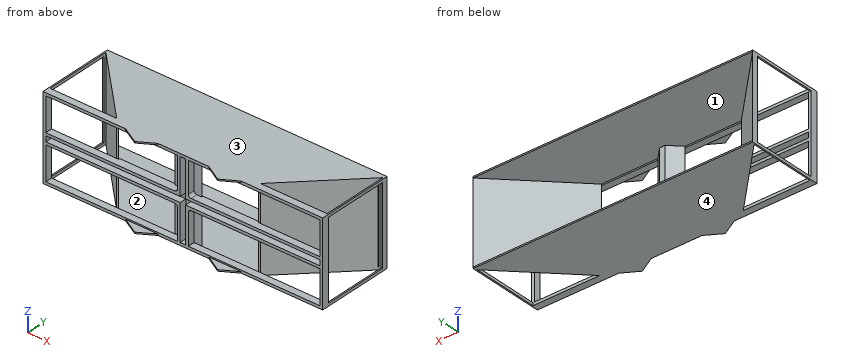
from build123d import *

# Parameters (mm, degrees)
BOSS_EXTRUDE1_DEPTH      = 10
BOSS_EXTRUDE1_DEPTH_BACK = 15
SKETCH1_W                = 1016
SKETCH1_H                = 304.8
SKETCH1_W_2              = 996
SKETCH1_H_2              = 284.8
BOSS_EXTRUDE2_DEPTH      = 10
BOSS_EXTRUDE2_DEPTH_BACK = 15
BOSS_EXTRUDE3_DEPTH      = 152.4
BOSS_EXTRUDE3_DEPTH_BACK = 152.4
SKETCH4_W                = 507.049279033
SKETCH4_H                = 40
BOSS_EXTRUDE7_DEPTH      = 5
SKETCH5_W                = 284.8
SKETCH5_H                = 234
CUT_EXTRUDE1_DEPTH       = 15
SKETCH6_W                = 284.8
SKETCH6_H                = 234
CUT_EXTRUDE2_DEPTH       = 15
BOSS_EXTRUDE8_DEPTH      = 304.8
BOSS_EXTRUDE9_DEPTH      = 5
BOSS_EXTRUDE10_DEPTH     = 5
BOSS_EXTRUDE11_DEPTH     = 5
BOSS_EXTRUDE12_DEPTH     = 5


with BuildPart() as part:
    # Sketch1 → Boss-Extrude1 (new, two sides: drawn at the far end of the back side and taken through both)
    with BuildSketch(Plane(origin=(0, 0, 0), x_dir=(1, 0, 0), z_dir=(0, 1, 0)).offset(-BOSS_EXTRUDE1_DEPTH_BACK)):
        Rectangle(SKETCH1_W, SKETCH1_H)
        Rectangle(SKETCH1_W_2, SKETCH1_H_2, mode=Mode.SUBTRACT)
    extrude(amount=BOSS_EXTRUDE1_DEPTH + BOSS_EXTRUDE1_DEPTH_BACK)

    # Sketch2 → Boss-Extrude2 (add, two sides: drawn at the far end of the back side and taken through both)
    with BuildSketch(Plane(origin=(0, 0, 0), x_dir=(1, 0, 0), z_dir=(0, 1, 0)).offset(-BOSS_EXTRUDE2_DEPTH_BACK)):
        with BuildLine():
            Line((-498, 20), (-30, 20))
            ThreePointArc((-30, 20), (-22.928932188, 22.928932188), (-20, 30))
            Line((-20, 30), (-20, 142.4))
            Line((-20, 142.4), (-10, 142.4))
            Line((-10, 142.4), (-10, 20))
            Line((-10, 20), (-10, 10))
            Line((-10, 10), (-498, 10))
            Line((-498, 10), (-498, 20))
        make_face()
        with BuildLine():
            Line((498, 20), (498, 10))
            Line((498, 10), (10, 10))
            Line((10, 10), (10, 20))
            Line((10, 20), (10, 142.4))
            Line((10, 142.4), (20, 142.4))
            Line((20, 142.4), (20, 30))
            ThreePointArc((20, 30), (22.928932188, 22.928932188), (30, 20))
            Line((30, 20), (498, 20))
        make_face()
        with BuildLine():
            Line((-498, -10), (-10, -10))
            Line((-10, -10), (-10, -20))
            Line((-10, -20), (-10, -142.4))
            Line((-10, -142.4), (-20, -142.4))
            Line((-20, -142.4), (-20, -30))
            ThreePointArc((-20, -30), (-22.928932188, -22.928932188), (-30, -20))
            Line((-30, -20), (-498, -20))
            Line((-498, -20), (-498, -10))
        make_face()
        with BuildLine():
            Line((30, -20), (498, -20))
            Line((498, -20), (498, -10))
            Line((498, -10), (10, -10))
            Line((10, -10), (10, -20))
            Line((10, -20), (10, -142.4))
            Line((10, -142.4), (20, -142.4))
            Line((20, -142.4), (20, -30))
            ThreePointArc((20, -30), (22.928932188, -22.928932188), (30, -20))
        make_face()
    extrude(amount=BOSS_EXTRUDE2_DEPTH + BOSS_EXTRUDE2_DEPTH_BACK)

    # Sketch3 → Boss-Extrude3 (add, two sides: drawn at the far end of the back side and taken through both)
    with BuildSketch(Plane.XY.offset(-BOSS_EXTRUDE3_DEPTH_BACK)):
        Polygon((-508, 10), (-508, 264), (-254, 10), (-261.071067812, 10), (-503, 251.928932188), (-503, 10), align=None)
        Polygon((261.071067812, 10), (254, 10), (508, 264), (508, 10), (503, 10), (503, 251.928932188), align=None)
    extrude(amount=BOSS_EXTRUDE3_DEPTH + BOSS_EXTRUDE3_DEPTH_BACK)

    # Sketch4 → Boss-Extrude7 (add)
    with BuildSketch(Plane(origin=(0, 10, 0), x_dir=(1, 0, 0), z_dir=(0, 1, 0))):
        with Locations((-0.42499269, 0)):
            Rectangle(SKETCH4_W, SKETCH4_H)
    extrude(amount=BOSS_EXTRUDE7_DEPTH)

    # Sketch5 → Cut-Extrude1 (cut)
    with BuildSketch(Plane(origin=(508, 0, 0), x_dir=(0, 0, -1), z_dir=(1, 0, 0))):
        with Locations((0, 127)):
            Rectangle(SKETCH5_W, SKETCH5_H)
    extrude(amount=-CUT_EXTRUDE1_DEPTH, mode=Mode.SUBTRACT)

    # Sketch6 → Cut-Extrude2 (cut)
    with BuildSketch(Plane.ZY.offset(508)):
        with Locations((0, 127)):
            Rectangle(SKETCH6_W, SKETCH6_H)
    extrude(amount=-CUT_EXTRUDE2_DEPTH, mode=Mode.SUBTRACT)

    # Sketch7 → Boss-Extrude8 (add)
    with BuildSketch(Plane(origin=(0, 0, -152.4), x_dir=(-1, 0, 0), z_dir=(0, 0, -1))):
        Polygon((-49.38581657, 10), (-9.847908285, 49.537908285), (10.152091715, 49.537908285), (49.69, 10), align=None)
    extrude(amount=-BOSS_EXTRUDE8_DEPTH)

    # Sketch8 → Boss-Extrude9 (add)
    with BuildSketch(Plane.XY.offset(152.4)):
        Polygon((-508, 264), (508, 264), (254, 10), (-254, 10), align=None)
    extrude(amount=-BOSS_EXTRUDE9_DEPTH)

    # Sketch9 → Boss-Extrude10 (add)
    with BuildSketch(Plane(origin=(0, 0, -152.4), x_dir=(-1, 0, 0), z_dir=(0, 0, -1))):
        Polygon((-508, 264), (508, 264), (254, 10), (-254, 10), align=None)
    extrude(amount=-BOSS_EXTRUDE10_DEPTH)

    # Sketch10 → Boss-Extrude11 (add)
    with BuildSketch(Plane.XY.offset(152.4)):
        Polygon((-254, 10), (-146.084980294, -48.838499263), (-49.69, 10), align=None)
        Polygon((49.38581657, 10), (155.071097682, -49.018715311), (254, 10), align=None)
    extrude(amount=-BOSS_EXTRUDE11_DEPTH)

    # Sketch11 → Boss-Extrude12 (add)
    with BuildSketch(Plane(origin=(0, 0, -152.4), x_dir=(-1, 0, 0), z_dir=(0, 0, -1))):
        Polygon((-212.094266455, -15), (-155.071097682, -49.018715311), (-94.153514645, -15), align=None)
        Polygon((90.647443469, -15), (146.084980294, -48.838499263), (208.147785439, -15), align=None)
    extrude(amount=-BOSS_EXTRUDE12_DEPTH)


solid = part.part
Read the model definition and answer for the solid it produces. Units are mm, in the model's axes. Face numbers are marked on the shaded views. Coordinates: 2 decimals unless noted, no trailing zeros. Loops run counter-clockwise (first coordinate to the right, second up) from the corner with the lowest first, then second, coordinate; pieces in that order, holes last. Notation, with made-up numbers: (60.5, 69.25) -> (89.5, 69.25) arc R21 ccw to (89.5, 83.25) -> close; hole circle Ø11 at (-27.5, -25.75). An arc over 180 degrees is marked (long way). Answer in a Markdown table with one row per item.
Item 1: A cutting plane is placed at B-B on y = 201.5. Determine the outline of the cut face in (x, z).
Returned:
| item | result |
|---|---|
| outline | (-508, -152.4) -> (-503, -152.4) -> (-503, -142.4) -> (-508, -142.4) -> close; (-508, 142.4) -> (-503, 142.4) -> (-503, 152.4) -> (-508, 152.4) -> close; (-452.57, -152.4) -> (452.57, -152.4) -> (452.57, 152.4) -> (-452.57, 152.4) -> close; (503, -152.4) -> (508, -152.4) -> (508, -142.4) -> (503, -142.4) -> close; (503, 142.4) -> (508, 142.4) -> (508, 152.4) -> (503, 152.4) -> close; hole (-445.5, -147.4) -> (445.5, -147.4) -> (445.5, 147.4) -> (-445.5, 147.4) -> close |
Item 2: A cutting plane is placed at D-D on y = 29. Determine the outline of the cut face in (x, z).
Returned:
| item | result |
|---|---|
| outline | (-508, -152.4) -> (-503, -152.4) -> (-503, -142.4) -> (-508, -142.4) -> close; (-508, 142.4) -> (-503, 142.4) -> (-503, 152.4) -> (-508, 152.4) -> close; (-280.07, -152.4) -> (280.07, -152.4) -> (280.07, 152.4) -> (-280.07, 152.4) -> close; (503, -152.4) -> (508, -152.4) -> (508, -142.4) -> (503, -142.4) -> close; (503, 142.4) -> (508, 142.4) -> (508, 152.4) -> (503, 152.4) -> close; hole (-273, -147.4) -> (-30.69, -147.4) -> (-30.69, 147.4) -> (-273, 147.4) -> close; hole (30.39, -147.4) -> (273, -147.4) -> (273, 147.4) -> (30.39, 147.4) -> close |
Item 3: A cutting plane is placed at A-A on x = 84.5. Determine the outline of the cut face in (y, z), plus the area to 3 significant figures.
Returned:
| item | result |
|---|---|
| outline | (-15, -152.4) -> (264, -152.4) -> (264, -147.4) -> (10, -147.4) -> (10, -142.4) -> (-15, -142.4) -> close; (-15, -20) -> (15, -20) -> (15, 20) -> (-15, 20) -> (-15, 10) -> (10, 10) -> (10, -10) -> (-15, -10) -> close; (-15, 142.4) -> (10, 142.4) -> (10, 147.4) -> (264, 147.4) -> (264, 152.4) -> (-15, 152.4) -> close |
| area | 3,740 mm^2 |
Item 4: A cutting plane is placed at C-C on x = 348.5. Determine the outline of the cut face in (y, z).
Returned:
| item | result |
|---|---|
| outline | (-15, -152.4) -> (10, -152.4) -> (10, -142.4) -> (-15, -142.4) -> close; (-15, -20) -> (10, -20) -> (10, -10) -> (-15, -10) -> close; (-15, 10) -> (10, 10) -> (10, 20) -> (-15, 20) -> close; (-15, 142.4) -> (10, 142.4) -> (10, 152.4) -> (-15, 152.4) -> close; (97.43, -152.4) -> (264, -152.4) -> (264, -147.4) -> (104.5, -147.4) -> (104.5, 147.4) -> (264, 147.4) -> (264, 152.4) -> (97.43, 152.4) -> close |
Item 5: Each of these flat-tipped pins is pushed along its axis until it touches: P1, Ø6, axis at y = 127, z = -67, coming from the -X side; P2, Ø3.5, axis at x = -256, z = -74.5, coming from the -Y side; P3, Ø12, axis at x = 152.5, z = 5, coming from the +Y side. Where does it stop, or does it pass through?
Returned:
| item | result |
|---|---|
| P1 | stops at x = -381.07 |
| P2 | stops at y = 10 |
| P3 | stops at y = 15 |
Item 6: For a pull along Z with two mould halves and no side action, classify the marked faces 1, 2, 3 and 4 as released by +Z, released by -Z, zero draft, split by the parting line, or undercut.
Returned:
| item | result |
|---|---|
| face 1 | undercut |
| face 2 | undercut |
| face 3 | released by +Z |
| face 4 | released by -Z |
Item 7: Straight lines are drawn through the part: line 1 along Z through (x, y) = (381.5, 144); line 2 along Z through (x, y) = (7, -2.5); line 3 along Z through (x, y) = (-427.5, -8). For each, find the intervals that lie inside material, in ascending order. Write a range as [from, to].
Returned:
| item | result |
|---|---|
| line 1 | z = [-152.4, -147.4], [147.4, 152.4] |
| line 2 | z = [-152.4, -142.4], [142.4, 152.4] |
| line 3 | z = [-152.4, -142.4], [-20, -10], [10, 20], [142.4, 152.4] |
